```python
from build123d import *

# Parameters (mm, degrees)
F1_DEPTH = 4.445
F2_R     = 2
F3_DEPTH = 4.446


with BuildPart() as f1:
    # F0 (on Front) → F1 (new body)
    with BuildSketch(Plane.XZ):
        with BuildLine():
            Line((-91.770717, 21.770717), (-71.770717, 21.770717))
            ThreePointArc((-71.770717, 21.770717), (-53.033009, 53.033009), (-21.770717, 71.770717))
            Line((-21.770717, 71.770717), (-21.770717, 91.770717))
            Line((-21.770717, 91.770717), (-91.770717, 91.770717))
            Line((-91.770717, 91.770717), (-91.770717, 21.770717))
        make_face()
        with BuildLine():
            ThreePointArc((-52.409953, 68.185019), (-60.811183, 60.811183), (-68.185019, 52.409953))
            ThreePointArc((-68.185019, 52.409953), (-70.41438, 51.735195), (-71.770717, 53.628789))
            Line((-71.770717, 53.628789), (-71.770717, 69.770717))
            ThreePointArc((-71.770717, 69.770717), (-71.184931, 71.184931), (-69.770717, 71.770717))
            Line((-69.770717, 71.770717), (-53.628789, 71.770717))
            ThreePointArc((-53.628789, 71.770717), (-51.735195, 70.41438), (-52.409953, 68.185019))
        make_face(mode=Mode.SUBTRACT)
    extrude(amount=F1_DEPTH)

    # F2 (on face) → F3 (cut, through all)
    with BuildSketch(Plane.XZ.offset(4.445)):
        with Locations((-63.270717, 81.770717)):
            Circle(F2_R)
        with Locations((-30.270717, 81.770717)):
            Circle(F2_R)
        with Locations((-81.770717, 63.270717)):
            Circle(F2_R)
        with Locations((-81.770717, 30.270717)):
            Circle(F2_R)
    extrude(amount=-F3_DEPTH, mode=Mode.SUBTRACT)


solid = f1.part
```
Check sheet for the modelled part. Datum: model origin and axes. Units: mm. A direction names the side the tool comes from. Coordinates: 2 decimals unless noted, no trailing zeros. Loops run counter-clockwise (first coordinate to the right, second up) from the corner with the lowest first, then second, coordinate; pieces in that order, holes last.
1) Material ranges on probe 1 along Z at (x, y) = (-80.5, -3.3); probe 2 along Z at (x, y) = (-62.5, -3.6); probe 3 along Z at (x, y) = (-53.5, -1.5), recorded low to high.
2) Sectioned sample at B-B (x = -29.5). Record the boundary of the cut face in (y, z) (3 decimals), and give its area (3 significant figures).
3) Sectioned sample at C-C (y = -3.25). Record the boundary of the cut face in (x, z), and give its area (3 significant figures).
4) Gauge pin test, flat end, axial feed: pin 1 (1 mm diameter, centred on x = -34.5, y = -3.5, fed in from -Z). Record the tip position at first contact, or that the pin passes through.
5) Release check for a two-part mould opening along X. For faces 3 (the face through (-82, -2, 21.771)), 4 (the face through (-91.771, -2, 57)), 5 (the face through (-21.771, -2, 82)), 6 (the face through (-83.245, -2.254, 31.622)) record: released by +X, released by -X, zero draft, split by the parting line, or undercut.
6) Sectioned sample at A-A (z = 59.5). Record the boundary of the cut face in (x, y) (3 decimals), and give its area (3 significant figures).
7) Sectioned sample at D-D (z = 42). Record the boundary of the cut face in (x, y) (3 decimals), and give its area (3 significant figures).
8) Access from +Z, -Z, +X, -X, +Y, -Y to the whole of each face (thin tool, end or side, straight path). Record for faces 1 (the face through (-71.771, -2, 62)), 2 (the face through (-53.396, -2.191, 52.667)).
Check sheet entries:
1. probe 1: z = 21.77 to 28.73, 31.82 to 61.73, 64.82 to 91.77
1. probe 2: z = 41.46 to 59.07, 71.77 to 79.93, 83.62 to 91.77
1. probe 3: z = 52.56 to 67.33, 71.77 to 91.77
2. outline: (-4.445, 68.955) - (0, 68.955) - (0, 79.925) - (-4.445, 79.925) - close; (-4.445, 83.616) - (0, 83.616) - (0, 91.771) - (-4.445, 91.771) - close
2. area: 85.0 mm2
3. outline: (-91.77, 21.77) - (-71.77, 21.77) arc R75 cw to (-21.77, 71.77) - (-21.77, 91.77) - (-91.77, 91.77) - close; hole circle Ø4 at (-81.77, 30.27); hole circle Ø4 at (-81.77, 63.27); hole (-71.77, 53.63) arc R2 ccw to (-68.19, 52.41) arc R86 cw to (-52.41, 68.19) arc R2 ccw to (-53.63, 71.77) - (-69.77, 71.77) arc R2 ccw to (-71.77, 69.77) - close; hole circle Ø4 at (-63.27, 81.77); hole circle Ø4 at (-30.27, 81.77)
3. area: 2,940 mm2
4. pin 1: stops at z = 66.33
5. face 3: zero draft
5. face 4: released by -X
5. face 5: released by +X
5. face 6: undercut
6. outline: (-91.771, -4.445) - (-71.771, -4.445) - (-71.771, 0) - (-91.771, 0) - close; (-62.095, -4.445) - (-45.659, -4.445) - (-45.659, 0) - (-62.095, 0) - close
6. area: 162 mm2
7. outline: (-91.771, -4.445) - (-62.137, -4.445) - (-62.137, 0) - (-91.771, 0) - close
7. area: 132 mm2
8. face 1: +Y, -Y
8. face 2: -Z, +X, +Y, -Y
